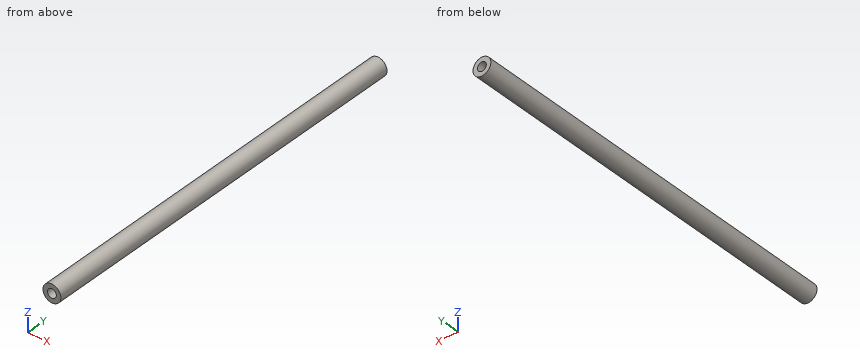
```python
from build123d import *

# Parameters (mm, degrees)
SKETCH1_R           = 4
BOSS_EXTRUDE1_DEPTH = 175
SKETCH2_R           = 2
CUT_EXTRUDE1_DEPTH  = 30


with BuildPart() as part:
    # Sketch1 → Boss-Extrude1 (new body)
    with BuildSketch(Plane(origin=(0, 0, 0), x_dir=(1, 0, 0), z_dir=(0, 1, 0))):
        with Locations(Location((0, 0, 0), (0, 0, 270))):
            Circle(SKETCH1_R)
    extrude(amount=BOSS_EXTRUDE1_DEPTH)

    # Sketch2 → Cut-Extrude1 (cut)
    with BuildSketch(Plane.XZ):
        with Locations(Location((0, 0, 0), (0, 0, 270))):
            Circle(SKETCH2_R)
    cut_extrude1 = extrude(amount=-CUT_EXTRUDE1_DEPTH, mode=Mode.SUBTRACT)

    # Mirror1: Cut-Extrude1 across plane
    add(cut_extrude1.mirror(Plane(origin=(0, 87.5, 0), x_dir=(0, 0, 1), z_dir=(0, -1, 0))), mode=Mode.SUBTRACT)


solid = part.part
```
Source: CAD feature listing. Evaluate the final solid. Frame: model axes, mm. Coordinates: 2 decimals unless noted, no trailing zeros. Loops run counter-clockwise (first coordinate to the right, second up) from the corner with the lowest first, then second, coordinate; pieces in that order, holes last. Notation, with made-up numbers: M 53,80 L 67,80 A24 cw 67,99 Z; hole C 7,-23 d2. An arc over 180 degrees is marked long. Use a Markdown table: item, result. Add a question column.
Q1. Material intervals for L1, parallel to Z at x = 0.25, y = 26; L2, parallel to X at y = 155, z = 0; L3, parallel to Y at x = -1, z = 0, sorted ascending.
Q2. Section query C-C, the plane y = 28. Return loops of the section in (x, z).
Q3. First-contact query: pin 1 (1.2 mm diameter, centred on x = 0.5, z = 0, fed in from +Y); pin 2 (4 mm diameter, centred on y = 131.5, z = 3, fed in from -X); pin 3 (1.2 mm diameter, centred on x = 0.5, z = 0.5, fed in from -Y). Flat tips, straight axial feed; report the tip coordinate or a pass-through.
Q4. Section query A-A, the plane z = 0. Return loops of the section in (x, y), and give its area (3 significant figures).
Q5. Section query B-B, the plane x = 0. Return loops of the section in (y, z), and give its area (3 significant figures).
Q6. Section query D-D, the plane y = 118. Return loops of the section in (x, z).
Result:
| question | item | result |
|---|---|---|
| 1 | L1 | z = -3.99 to -1.98, 1.98 to 3.99 |
| 1 | L2 | x = -4 to -2, 2 to 4 |
| 1 | L3 | y = 30 to 145 |
| 2 | outline | C 0,0 d8; hole C 0,0 d4 |
| 3 | pin 1 | stops at y = 145 |
| 3 | pin 2 | stops at x = -3.87 |
| 3 | pin 3 | stops at y = 30 |
| 4 | outline | M -4,0 L -2,0 L -2,30 L 2,30 L 2,0 L 4,0 L 4,175 L 2,175 L 2,145 L -2,145 L -2,175 L -4,175 Z |
| 4 | area | 1,160 mm2 |
| 5 | outline | M 0,-4 L 175,-4 L 175,-2 L 145,-2 L 145,2 L 175,2 L 175,4 L 0,4 L 0,2 L 30,2 L 30,-2 L 0,-2 Z |
| 5 | area | 1,160 mm2 |
| 6 | outline | C 0,0 d8 |
